from build123d import *

# Parameters (mm, degrees)
SKETCH1_W                   = 70
SKETCH1_H                   = 290
BASE_FLANGE1_DEPTH          = 3
SM_EDGE_FLANGE_1_DEPTH      = 290
SM_EDGE_FLANGE_1_BEND_DEPTH = 290
INDENT1_START               = -127
INDENT1_DEPTH               = 84
INDENT1_START_2             = -123.729611107
INDENT1_2_DEPTH             = 77.459222009
INDENT1_3_DEPTH             = 0.729611107
INDENT1_START_3             = -47
INDENT1_4_DEPTH             = 0.729610902
INDENT1_START_4             = -50.0000001
INDENT1_5_DEPTH             = 6.0000001
INDENT1_START_5             = -126
INDENT1_6_DEPTH             = 6
INDENT1_START_6             = -290
INDENT1_7_DEPTH             = 6.65
INDENT2_START               = -127
INDENT2_DEPTH               = 84
INDENT2_START_2             = -11.0000001
INDENT2_2_DEPTH             = 11.0000001
INDENT2_START_3             = -126
INDENT2_3_DEPTH             = 82
CUT_EXTRUDE1_DEPTH          = 317.754179273
CUT_EXTRUDE1_DEPTH_BACK     = 317.754179273
SKETCH12_R                  = 4.2
CUT_EXTRUDE2_DEPTH          = 10


with BuildPart() as part:
    # Base-Flange1: sheet metal written as solids
    # Sketch1 → Base-Flange1 (new body)
    with BuildSketch(Plane(origin=(0, 207.95, 0), x_dir=(1, 0, 0), z_dir=(0, 1, 0))):
        with Locations((-85, 145)):
            Rectangle(SKETCH1_W, SKETCH1_H)
    extrude(amount=-BASE_FLANGE1_DEPTH)

    # 邊線-凸緣1: sheet metal written as solids
    # 邊線-凸緣1 section (on a plane across the edge) → 邊線-凸緣1 (add)
    with BuildSketch(Plane(origin=(-47, 204.95, -290), x_dir=(-1, 0, 0), z_dir=(0, 0, 1))):
        with BuildLine():
            Line((-3, 3), (-3, 15.9))
            Line((-3, 15.9), (0, 15.9))
            Line((0, 15.9), (0, 3))
            ThreePointArc((0, 3), (0.878679656, 0.878679656), (3, 0))
            Line((3, 0), (3, -3))
            ThreePointArc((3, -3), (-1.242640687, -1.242640687), (-3, 3))
        make_face()
    extrude(amount=SM_EDGE_FLANGE_1_DEPTH)

    # 邊線-凸緣1 section 2 (on a plane across the edge) → 邊線-凸緣1 bend (add)
    with BuildSketch(Plane(origin=(-123, 204.95, 0), x_dir=(1, 0, 0), z_dir=(0, 0, -1))):
        with BuildLine():
            Line((-3, 3), (-3, 15.9))
            Line((-3, 15.9), (0, 15.9))
            Line((0, 15.9), (0, 3))
            ThreePointArc((0, 3), (0.878679656, 0.878679656), (3, 0))
            Line((3, 0), (3, -3))
            ThreePointArc((3, -3), (-1.242640687, -1.242640687), (-3, 3))
        make_face()
    extrude(amount=SM_EDGE_FLANGE_1_BEND_DEPTH)

    # Indent1: read off the stored shape, not the designer's step
    # Indent1 outline → Indent1 (cut)
    with BuildSketch(Plane.YZ.offset(INDENT1_START)):
        with BuildLine():
            Line((192.05, -290), (207.95, -290))
            ThreePointArc((207.95, -290), (200, -282.05), (192.05, -290))
        make_face()
    extrude(amount=INDENT1_DEPTH, mode=Mode.SUBTRACT)

    # Indent2: read off the stored shape, not the designer's step
    # Indent2 outline → Indent2 (cut)
    with BuildSketch(Plane.YZ.offset(INDENT2_START)):
        with BuildLine():
            ThreePointArc((189.05, -6.433311744), (197.7062633, -12.491147744), (207.950014124, -9.903902031))
            Line((207.950014124, -9.903902031), (209, -9.061062257))
            Line((209, -9.061062257), (209, 1))
            Line((209, 1), (188, 1))
            Line((188, 1), (188, 0))
            Line((188, 0), (188, -4.64612958))
            Line((188, -4.64612958), (189.05, -6.433311744))
        make_face()
    extrude(amount=INDENT2_DEPTH, mode=Mode.SUBTRACT)

    # Sketch12 → Cut-Extrude1 (cut, two sides: drawn at the far end of the back side and taken through both)
    with BuildSketch(Plane(origin=(0, 207.95, 0), x_dir=(1, 0, 0), z_dir=(0, 1, 0)).offset(-CUT_EXTRUDE1_DEPTH_BACK)):
        with Locations((-109.5, 270.8)):
            Circle(SKETCH12_R)
        with Locations((-60.5, 270.8)):
            Circle(SKETCH12_R)
        with Locations((-60.5, 250.8)):
            Circle(SKETCH12_R)
        with Locations((-109.5, 250.8)):
            Circle(SKETCH12_R)
        with Locations((-60.5, 230.8)):
            Circle(SKETCH12_R)
        with Locations((-109.5, 230.8)):
            Circle(SKETCH12_R)
        with Locations((-60.5, 210.8)):
            Circle(SKETCH12_R)
        with Locations((-109.5, 210.8)):
            Circle(SKETCH12_R)
        with Locations((-60.5, 190.8)):
            Circle(SKETCH12_R)
        with Locations((-109.5, 190.8)):
            Circle(SKETCH12_R)
        with Locations((-60.5, 170.8)):
            Circle(SKETCH12_R)
        with Locations((-109.5, 170.8)):
            Circle(SKETCH12_R)
        with Locations((-60.5, 150.8)):
            Circle(SKETCH12_R)
        with Locations((-109.5, 150.8)):
            Circle(SKETCH12_R)
        with Locations((-60.5, 130.8)):
            Circle(SKETCH12_R)
        with Locations((-109.5, 130.8)):
            Circle(SKETCH12_R)
        with Locations((-60.5, 110.8)):
            Circle(SKETCH12_R)
        with Locations((-109.5, 110.8)):
            Circle(SKETCH12_R)
    extrude(amount=CUT_EXTRUDE1_DEPTH + CUT_EXTRUDE1_DEPTH_BACK, mode=Mode.SUBTRACT)

    # Sketch13 → Cut-Extrude2 (cut)
    with BuildSketch(Plane(origin=(0, 207.95, 0), x_dir=(1, 0, 0), z_dir=(0, 1, 0))):
        with BuildLine():
            Line((-70, 107.7), (-70, 42.7))
            ThreePointArc((-70, 42.7), (-85, 27.7), (-100, 42.7))
            Line((-100, 42.7), (-100, 107.7))
            ThreePointArc((-100, 107.7), (-85, 122.7), (-70, 107.7))
        make_face()
    extrude(amount=-CUT_EXTRUDE2_DEPTH, mode=Mode.SUBTRACT)


with BuildPart() as body_2:
    # Indent1 2 outline → Indent1 2 (new body)
    with BuildSketch(Plane.YZ.offset(INDENT1_START_2)):
        with BuildLine():
            Line((204.95, -285.559279338), (204.95, -290))
            Line((204.95, -290), (206.65, -290))
            ThreePointArc((206.65, -290), (206.210475022, -287.622501314), (204.95, -285.559279338))
        make_face()
    extrude(amount=INDENT1_2_DEPTH)

    # Indent1 3 outline → Indent1 3 (add)
    with BuildSketch(Plane.YZ.offset(INDENT1_START_2)):
        with BuildLine():
            Line((193.35, -290), (204.95, -290))
            Line((204.95, -290), (204.95, -285.559279338))
            ThreePointArc((204.95, -285.559279338), (197.622501314, -283.789524978), (193.35, -290))
        make_face()
    extrude(amount=INDENT1_3_DEPTH)

    # Indent1 4 outline → Indent1 4 (add)
    with BuildSketch(Plane.YZ.offset(INDENT1_START_3)):
        with BuildLine():
            Line((193.35, -290), (204.95, -290))
            Line((204.95, -290), (204.95, -285.559279338))
            ThreePointArc((204.95, -285.559279338), (197.622501314, -283.789524978), (193.35, -290))
        make_face()
    extrude(amount=INDENT1_4_DEPTH)

    # Indent1 5 outline → Indent1 5 (add)
    with BuildSketch(Plane.YZ.offset(INDENT1_START_4)):
        with BuildLine():
            Line((193.35, -290), (206.65, -290))
            ThreePointArc((206.65, -290), (200, -283.35), (193.35, -290))
        make_face()
    extrude(amount=INDENT1_5_DEPTH)

    # Indent1 6 outline → Indent1 6 (add)
    with BuildSketch(Plane.YZ.offset(INDENT1_START_5)):
        with BuildLine():
            Line((193.35, -290), (206.65, -290))
            ThreePointArc((206.65, -290), (200, -283.35), (193.35, -290))
        make_face()
    extrude(amount=INDENT1_6_DEPTH)

    # Indent1 7 outline → Indent1 7 (cut)
    with BuildSketch(Plane.XY.offset(INDENT1_START_6)):
        with BuildLine():
            Line((-47, 192), (-47, 201.95))
            ThreePointArc((-47, 201.95), (-47.878679656, 204.071320344), (-50, 204.95))
            Line((-50, 204.95), (-50.0000001, 192))
            Line((-50.0000001, 192), (-47, 192))
        make_face()
        with BuildLine():
            Line((-123, 192), (-120, 192))
            Line((-120, 192), (-120, 204.95))
            ThreePointArc((-120, 204.95), (-122.121320344, 204.071320344), (-123, 201.95))
            Line((-123, 201.95), (-123, 192))
        make_face()
        with BuildLine():
            ThreePointArc((-46.270396534, 206.650006169), (-44.597333029, 204.559825589), (-44, 201.95))
            Line((-44, 201.95), (-44, 208))
            Line((-44, 208), (-47.971644239, 208))
            Line((-47.971644239, 208), (-46.270396534, 206.650006169))
        make_face()
        with BuildLine():
            Line((-126, 208), (-126, 201.95))
            ThreePointArc((-126, 201.95), (-125.402668364, 204.559822705), (-123.729608483, 206.650002187))
            Line((-123.729608483, 206.650002187), (-122.028359489, 208))
            Line((-122.028359489, 208), (-126, 208))
        make_face()
    extrude(amount=INDENT1_7_DEPTH, mode=Mode.SUBTRACT)


with BuildPart() as body_3:
    # Indent2 2 outline → Indent2 2 (new body)
    with BuildSketch(Plane.XY.offset(INDENT2_START_2)):
        with BuildLine():
            Line((-44, 189.05), (-44, 201.95))
            ThreePointArc((-44, 201.95), (-45.757359313, 206.192640687), (-50, 207.95))
            Line((-50, 207.95), (-120, 207.95))
            ThreePointArc((-120, 207.95), (-124.242640687, 206.192640687), (-126, 201.95))
            Line((-126, 201.95), (-126, 189.05))
            Line((-126, 189.05), (-123, 189.05))
            Line((-123, 189.05), (-123, 201.95))
            ThreePointArc((-123, 201.95), (-122.121320344, 204.071320344), (-120, 204.95))
            Line((-120, 204.95), (-50, 204.95))
            ThreePointArc((-50, 204.95), (-47.878679656, 204.071320344), (-47, 201.95))
            Line((-47, 201.95), (-47, 189.05))
            Line((-47, 189.05), (-44, 189.05))
        make_face()
    extrude(amount=INDENT2_2_DEPTH)

    # Indent2 3 outline → Indent2 3 (cut)
    with BuildSketch(Plane.YZ.offset(INDENT2_START_3)):
        with BuildLine():
            Line((207.95, -11.0000001), (207.950016725, -7.602449216))
            ThreePointArc((207.950016725, -7.602449216), (204.322791843, -10.115012145), (200.000000001, -11))
            Line((200.000000001, -11), (207.95, -11.0000001))
        make_face()
        with BuildLine():
            Line((189.05, -11.0000001), (200.000000001, -11))
            ThreePointArc((200.000000001, -11), (192.601479194, -8.140140655), (189.05, -1.047616342))
            Line((189.05, -1.047616342), (189.05, -11.0000001))
        make_face()
    extrude(amount=INDENT2_3_DEPTH, mode=Mode.SUBTRACT)


solid = part.part
The model under review builds one solid part; all positions refer to its coordinate system, in mm. A direction names the side the tool comes from. Round coordinates to 2 decimals unless told otherwise and drop trailing zeros. Loops run counter-clockwise (first coordinate to the right, second up) from the corner with the lowest first, then second, coordinate; pieces in that order, holes last. Notation, with made-up numbers: (-33, 42.25) -> (9, 42.25) arc R20 cw to (9, 56.25) -> close; hole circle Ø5 at (61.25, 59.25). An arc over 180 degrees is marked (long way). One line per question, with ' | ' between items. Start each with the question number.
Item 1: Add section A-A, the plane z = -270.8. Write out the cut boundary in (x, y).
Item 2: Add section C-C, the plane x = -60.5. Count the separate pieces of the cut face and the enclosed holes in it, then the cut area to 3 significant figures.
Item 3: For pin 1 (9.5 mm diameter, centred on x = -60.5, z = -250.8, fed in from -Y); pin 2 (2.5 mm diameter, centred on y = 205.5, z = -82, fed in from +X); pin 3 (12 mm diameter, centred on x = -115.5, z = -177.5, fed in from -Y), all flat-tipped, find the tip position at first contact; note any pin that passes through.
Item 4: Draft analysis for pull direction X (two halves, no side actions). For faces 3 (the face through (-45.804, 206.239, -151.913)), 4 (the face through (-85.33, 206.471, -122.696)), state which applies: +X half, -X half, draft (parallel to the pull), parting line (faces both ways), or undercut.
Item 5: Machinability: for faces 1 (the face through (-63.596, 206.429, -273.639)), 2 (the face through (-123, 195, -146)), which of the approach directions +Z, -Z, +X, -X, +Y, -Y give a long, thin tool a straight path to every point of the face, cutting with its end or side? Answer none if there is none.
Item 6: Add section B-B, the plane z = -103. Write out the cut boundary in (x, y), then the cut area to 3 significant figures.
Item 7: Wall thickness on line 1 along X through (y, z) = (193.25, -126); line 2 along X through (y, z) = (206.2, -270.8); line 3 along Y through (x, z) = (-78.5, -192): over which ranges is each line inside the solid? List them lowest first. Write a range as [from, to].
Return value:
1) outline: (-126, 189.05) -> (-123, 189.05) -> (-123, 201.95) arc R3 cw to (-120, 204.95) -> (-113.7, 204.95) -> (-113.7, 207.95) -> (-120, 207.95) arc R6 ccw to (-126, 201.95) -> close; (-105.3, 204.95) -> (-64.7, 204.95) -> (-64.7, 207.95) -> (-105.3, 207.95) -> close; (-56.3, 204.95) -> (-50, 204.95) arc R3 cw to (-47, 201.95) -> (-47, 189.05) -> (-44, 189.05) -> (-44, 201.95) arc R6 ccw to (-50, 207.95) -> (-56.3, 207.95) -> close
2) separate pieces: 10 | enclosed holes: 0 | area: 598 mm2
3) pin 1: stops at y = 204.95 | pin 2: stops at x = -44.46 | pin 3: stops at y = 204.55
4) face 3: +X half | face 4: undercut
5) face 1: +Y, -Y | face 2: +Z, -Z, -Y
6) outline: (-126, 189.05) -> (-123, 189.05) -> (-123, 201.95) arc R3 cw to (-120, 204.95) -> (-100, 204.95) -> (-100, 207.95) -> (-120, 207.95) arc R6 ccw to (-126, 201.95) -> close; (-70, 204.95) -> (-50, 204.95) arc R3 cw to (-47, 201.95) -> (-47, 189.05) -> (-44, 189.05) -> (-44, 201.95) arc R6 ccw to (-50, 207.95) -> (-70, 207.95) -> close | area: 240 mm2
7) line 1: x = [-126, -123], [-47, -44] | line 2: x = [-124.24, -113.7], [-105.3, -64.7], [-56.3, -45.76] | line 3: y = [204.95, 207.95]
